```python
from build123d import *

# Parameters (mm, degrees)
EXTRUDE_1_DEPTH     = 83
EXTRUDE_START       = 3
SKETCH_2_R          = 5
EXTRUDE_2_DEPTH     = 4.4
SKETCH_3_R          = 1.6
CUT_EXTRUDE_1_DEPTH = 7.4
CHAMFER_1_SIZE      = 2
SKETCH_4_W          = 9
SKETCH_4_H          = 3
SKETCH_4_W_2        = 3
SKETCH_4_H_2        = 9
EXTRUDE_3_DEPTH     = 3
CHAMFER_2_SIZE      = 1
FILLET_1_R          = 2


with BuildPart() as part:
    # 草图1 → 凸台-拉伸1 (new, symmetric)
    with BuildSketch(Plane(origin=(0, 0, 0), x_dir=(0, 0, -1), z_dir=(1, 0, 0))):
        Polygon((0, 3), (0, 0), (95.8, 0), (92.8, 3), align=None)
    extrude(amount=EXTRUDE_1_DEPTH, both=True)

    # 草图2 → 凸台-拉伸2 (add)
    with BuildSketch(Plane(origin=(0, 0, 0), x_dir=(1, 0, 0), z_dir=(0, 1, 0)).offset(EXTRUDE_START)):
        with Locations(Location((-74, 9, 0), (0, 0, 90))):
            Circle(SKETCH_2_R)
        with Locations(Location((74, 9, 0), (0, 0, 90))):
            Circle(SKETCH_2_R)
        with Locations(Location((0, 65, 0), (0, 0, 90))):
            Circle(SKETCH_2_R)
        with Locations(Location((0, 31, 0), (0, 0, 90))):
            Circle(SKETCH_2_R)
    extrude(amount=EXTRUDE_2_DEPTH)

    # 草图3 → 切除-拉伸1 (cut)
    with BuildSketch(Plane(origin=(0, 0, 0), x_dir=(1, 0, 0), z_dir=(0, 1, 0))):
        with Locations(Location((74, 9, 0), (0, 0, 90))):
            Circle(SKETCH_3_R)
        with Locations(Location((-74, 9, 0), (0, 0, 90))):
            Circle(SKETCH_3_R)
        with Locations(Location((0, 65, 0), (0, 0, 90))):
            Circle(SKETCH_3_R)
    extrude(amount=CUT_EXTRUDE_1_DEPTH, mode=Mode.SUBTRACT)

    # 倒角1
    chamfer_1_edges = [part.edges().sort_by_distance(p)[0] for p in [
        (74, 0, -7.4),
        (-74, 0, -7.4),
        (0, 0, -63.4),
    ]]
    chamfer(chamfer_1_edges, length=CHAMFER_1_SIZE)

    # 草图4 → 凸台-拉伸3 (add)
    with BuildSketch(Plane(origin=(0, 0, 0), x_dir=(1, 0, 0), z_dir=(0, 1, 0)).offset(EXTRUDE_START)):
        with Locations((45.5, 4.5)):
            Rectangle(SKETCH_4_W, SKETCH_4_H)
        with Locations((-45.5, 4.5)):
            Rectangle(SKETCH_4_W, SKETCH_4_H)
        with Locations((-78.5, 60.5)):
            Rectangle(SKETCH_4_W_2, SKETCH_4_H_2)
        with Locations((78.5, 60.5)):
            Rectangle(SKETCH_4_W_2, SKETCH_4_H_2)
    extrude(amount=EXTRUDE_3_DEPTH)

    # 倒角2
    chamfer_2_edges = [part.edges().sort_by_distance(p)[0] for p in [
        (-74, 3, -4),
        (74, 3, -4),
        (0, 3, -60),
        (0, 3, -26),
    ]]
    chamfer(chamfer_2_edges, length=CHAMFER_2_SIZE)

    # 圆角1
    # the kernel refuses this fillet: 2 mm, written as the material it takes off along each edge
    with BuildSketch(Plane(origin=(-94.830127019, 0, -95.8), x_dir=(0, 0.7071067811865416, 0.7071067811865535), z_dir=(1, 0, 0))) as fillet_1_piece_1:
        with BuildLine():
            CenterArc((4.760278777, 1.931851653), FILLET_1_R, 135, 120)
            Line((3.346065215, 3.346065215), (3.317780944, 3.374349486))
            Line((3.317780944, 3.374349486), (-0.028284271, 0.028284271))
            Line((-0.028284271, 0.028284271), (0, -0.04))
            ThreePointArc((0, -0.04), (2.121320344, -0.04), (4.232287925, -0.038637033))
            Line((4.232287925, -0.038637033), (4.242640687, 0))
        make_face()
    extrude(amount=189.660254038, mode=Mode.SUBTRACT)


solid = part.part
```
Input: part model. Units: mm. Frame: model coordinates. A direction names the side the tool comes from. Round coordinates to 2 decimals unless told otherwise and drop trailing zeros. Loops run counter-clockwise (first coordinate to the right, second up) from the corner with the lowest first, then second, coordinate; pieces in that order, holes last.
1) Section query C-C on z = -31. Return the cut outline in (x, y), plus the area to 3 significant figures.
Ans:
outline: (-83, 0) - (83, 0) - (83, 3) - (6, 3) - (5, 4) - (5, 7.4) - (-5, 7.4) - (-5, 4) - (-6, 3) - (-83, 3) - close
area: 543 mm2
2) Section query B-B on x = 0. Return the cut outline in (y, z), plus the area to 3 significant figures.
Ans:
outline: (0, -91.07) arc R2 ccw to (3, -92.8) - (3, -71) - (4, -70) - (7.4, -70) - (7.4, -66.6) - (2, -66.6) - (0, -68.6) - close; (0, -61.4) - (2, -63.4) - (7.4, -63.4) - (7.4, -60) - (4, -60) - (3, -59) - (3, -37) - (4, -36) - (7.4, -36) - (7.4, -26) - (4, -26) - (3, -25) - (3, 0) - (0, 0) - close
area: 341 mm2
3) Set-up query: faces 1 (the flat face through (-79, 6, -61)), 2 (the flat face through (-80, 4, -60)), 3 (the flat face through (-77, 4, -60)), 4 (the cylindrical face through (0, 6, -26)). Return all of +Z, -Z, +X, -X, +Y, -Y with unobstructed straight access to the full face (end or side cutting, diameter ignored); none if empty.
Ans:
face 1: -Z, -X, +Y
face 2: +Z, -Z, -X, +Y
face 3: -Z, +Y
face 4: +Y
4) Pull-direction query (Z, two-part tool) for faces 5 (the flat face through (45, 4, -3)), 6 (the cylindrical face through (72.414, 4.662, -8.792)), 7 (the flat face through (78, 6, -61)); classes: released by +Z, released by -Z, zero draft, split by the parting line, or undercut.
Ans:
face 5: released by +Z
face 6: undercut
face 7: zero draft
5) Section query D-D on x = -17.5. Return the cut outline in (y, z), plus the area to 3 significant figures.
Ans:
outline: (0, -91.07) arc R2 ccw to (3, -92.8) - (3, 0) - (0, 0) - close
area: 278 mm2
6) Section query A-A on z = -9. Return the cut outline in (x, y).
Ans:
outline: (-83, 0) - (-77.6, 0) - (-75.6, 2) - (-75.6, 7.4) - (-79, 7.4) - (-79, 4) - (-80, 3) - (-83, 3) - close; (-72.4, 2) - (-70.4, 0) - (70.4, 0) - (72.4, 2) - (72.4, 7.4) - (69, 7.4) - (69, 4) - (68, 3) - (-68, 3) - (-69, 4) - (-69, 7.4) - (-72.4, 7.4) - close; (75.6, 2) - (77.6, 0) - (83, 0) - (83, 3) - (80, 3) - (79, 4) - (79, 7.4) - (75.6, 7.4) - close
7) Pin query (flat end, axial travel): pin 1 (3.5 mm diameter, centred on x = -47, y = 5, fed in from -Z); pin 2 (3 mm diameter, centred on x = -74, z = -9, fed in from -Y); pin 3 (1.5 mm diameter, centred on y = 4, z = -60, fed in from -X); pin 4 (0.9 mm diameter, centred on y = 4.5, z = -4.5, fed in from +X). Return the tip coordinate at first contact, or that it passes through.
Ans:
pin 1: stops at z = -6
pin 2: passes through
pin 3: stops at x = -80
pin 4: stops at x = 76.93
8) Material intervals for line 1 (X direction, y = 5, z = -62); line 2 (X direction, y = 5.45, z = -9); line 3 (Z direction, x = 74, y = 6.05), sorted ascending.
Ans:
line 1: x = -80 to -77, -4 to 4, 77 to 80
line 2: x = -79 to -75.6, -72.4 to -69, 69 to 72.4, 75.6 to 79
line 3: z = -14 to -10.6, -7.4 to -4
